The model under review builds one solid part; all positions refer to its coordinate system, in mm. Coordinates: 2 decimals unless noted, no trailing zeros. Write each loop counter-clockwise with the first axis right and the second up, starting at its lowest first coordinate (ties: lowest second). Pieces come first, ordered by that corner, then holes. Notation, with made-up numbers: (72.25, 36) -> (98.25, 36) arc R31 cw to (98.25, 61) -> close; hole circle Ø11 at (46, 34.25). An arc over 180 degrees is marked (long way). Put each result on its own line as item: value. Start each with the question number.
from build123d import *

# Parameters (mm, degrees)
F1_DEPTH = 19.05
F2_R     = 6.35
F2_R_2   = 12.7
F3_DEPTH = 50.8


with BuildPart() as f1:
    # F0 (on Front) → F1 (new body)
    with BuildSketch(Plane.XZ):
        with BuildLine():
            ThreePointArc((-12.7, 50.8), (-23.358147, 23.358147), (-50.8, 12.7))
            ThreePointArc((-50.8, 12.7), (-63.5, 0), (-50.8, -12.7))
            ThreePointArc((-50.8, -12.7), (-23.136197, -23.283192), (-12.421733, -50.896417))
            ThreePointArc((-12.421733, -50.896417), (0.180683, -61.674015), (12.7, -50.8))
            ThreePointArc((12.7, -50.8), (23.358147, -23.358147), (50.8, -12.7))
            ThreePointArc((50.8, -12.7), (63.5, 0), (50.8, 12.7))
            ThreePointArc((50.8, 12.7), (23.358147, 23.358147), (12.7, 50.8))
            ThreePointArc((12.7, 50.8), (0, 63.5), (-12.7, 50.8))
        make_face()
    extrude(amount=F1_DEPTH)

    # F2 (on Front) → F3 (cut)
    with BuildSketch(Plane.XZ):
        with Locations((0, 50.8)):
            Circle(F2_R)
        with Locations((50.8, 0)):
            Circle(F2_R)
        with Locations((0, -50.8)):
            Circle(F2_R)
        with Locations((-50.8, 0)):
            Circle(F2_R)
        Circle(F2_R_2)
    extrude(amount=F3_DEPTH, mode=Mode.SUBTRACT)


solid = f1.part
1. Wall thickness on line 1 (X direction, y = -10.75, z = 0); line 2 (Z direction, x = 0, y = -9); line 3 (X direction, y = -8.5, z = 50.8): over which ranges is each line inside the solid? List them lowest first. Write a range as from..to.
2. The part is to be moulded in two halves that separate along Z. For faces 1 (the cylindrical face through (-63.497, -9.392, 0.279)), 2 (the cylindrical face through (-0.072, -9.392, -61.672)), 3 (the cylindrical face through (-0.8, -9.4, 57.1)), say which applies: released by +Z, released by -Z, zero draft, split by the parting line, or undercut.
3. Consider section C-C on x = 0. State the section outline as (y, z) points.
4. Consider section B-B on y = -7.75. State how many separate pieces and enclosed holes the cut face has, then the cut area to 3 significant figures.
5. Consider section A-A on z = 0. State the section outline as (x, y) points, then the cut area to 3 significant figures.
6. Insertion check: P1, Ø1, axis at x = -30.5, y = -14, coming from the +Z side; P2, Ø3, axis at x = -34.5, y = -7.5, coming from the -Z side; P3, Ø10, axis at y = -12.5, z = -44, coming from the -X side; P4, Ø10, axis at x = 0, z = 50.8, coming from the +Y side. Each pin has a flat end and moves straight along its axis. Give the tip position at first contact, or say it passes through.
7. Consider section D-D on x = 27. State the section outline as (y, z) points.
Output values:
1. line 1: x = -63.5..-57.15, -44.45..-12.7, 12.7..44.45, 57.15..63.5
1. line 2: z = -61.67..-57.15, -44.45..-12.7, 12.7..44.45, 57.15..63.5
1. line 3: x = -12.7..-6.35, 6.35..12.7
2. face 1: split by the parting line
2. face 2: released by -Z
2. face 3: undercut
3. outline: (-19.05, -61.67) -> (0, -61.67) -> (0, -57.15) -> (-19.05, -57.15) -> close; (-19.05, -44.45) -> (0, -44.45) -> (0, -12.7) -> (-19.05, -12.7) -> close; (-19.05, 12.7) -> (0, 12.7) -> (0, 44.45) -> (-19.05, 44.45) -> close; (-19.05, 57.15) -> (0, 57.15) -> (0, 63.5) -> (-19.05, 63.5) -> close
4. separate pieces: 1
4. enclosed holes: 5
4. area: 5,590 mm^2
5. outline: (-63.5, -19.05) -> (-57.15, -19.05) -> (-57.15, 0) -> (-63.5, 0) -> close; (-44.45, -19.05) -> (-12.7, -19.05) -> (-12.7, 0) -> (-44.45, 0) -> close; (12.7, -19.05) -> (44.45, -19.05) -> (44.45, 0) -> (12.7, 0) -> close; (57.15, -19.05) -> (63.5, -19.05) -> (63.5, 0) -> (57.15, 0) -> close
5. area: 1,450 mm^2
6. P1: stops at z = 18.11
6. P2: stops at z = -16.29
6. P3: stops at x = -13.82
6. P4: passes through
7. outline: (-19.05, -20.17) -> (0, -20.17) -> (0, 20.17) -> (-19.05, 20.17) -> close
